Input: part model. Units: mm. Frame: model coordinates. Give positions to 0.01 mm unless a question says otherwise; leave off trailing zeros. Loops run counter-clockwise (first coordinate to the right, second up) from the corner with the lowest first, then second, coordinate; pieces in that order, holes last. Notation, with made-up numbers: (-5, 65.5) -> (47, 65.5) arc R24 ccw to (47, 104.5) -> close; hole circle Ø2 at (34.25, 36.25). An arc over 180 degrees is marked (long way). Answer as a JSON object with one key per item and string values.
Autodesk Inventor part; units mm, degrees
ref_plane "YZ Plane" through (0, 0, 0) normal (1, 0, 0) x (0, 1, 0)
ref_plane "XZ Plane" through (0, 0, 0) normal (0, 1, 0) x (-1, 0, 0)
ref_plane "XY Plane" through (0, 0, 0) normal (0, 0, 1) x (1, 0, 0)
sketch "Sketch1" plane through (0, 0, 0) normal (0, 1, 0) x (-1, 0, 0)
  line L0 (0, 0) -> (7.5, 0)
  line L1 (7.5, -18) -> (0, -18)
  line L2 (0, -18) -> (0, 0)
  arc A0 (7.5, -5) -> (7.5, -13) centre (7.5, -9) ccw
  line L3 (7.5, -18) -> (7.5, -13)
  line L4 (7.5, -5) -> (7.5, 0)
  dimension "d0" = 7.5
  dimension "d1" = 18
  dimension "d5" = 4
  dimension "d6" = 0
  dimension "d7" = 5
  dimension "d8" = 0
extrude "Extrusion2" add sketch "Sketch1" along normal blind 16
properties part number "Lower Base Bearing Holder" material "Brass, Soft Yellow"
Q1. Section D-D, the plane x = -7. Return the cut outline in (y, z), then the cut area to 3 significant figures.
Evaluation:
{"outline": "(0, -18) -> (16, -18) -> (16, -12.97) -> (0, -12.97) -> close; (0, -5.03) -> (16, -5.03) -> (16, 0) -> (0, 0) -> close", "area": "161 mm2"}
Q2. Draft query along Z for faces 1 (the cylindrical face through (-3.5, 7.9, -9.1)), 2 (the flat face through (-7.5, 8, -3)), 3 (the flat face through (-4, 8, -18)). Return one class per face: +Z half, -Z half, draft (parallel to the pull), parting line (faces both ways), or undercut.
Evaluation:
{"face 1": "undercut", "face 2": "draft", "face 3": "-Z half"}
Q3. Pin query (flat end, axial travel): pin 1 (4 mm diameter, centred on y = 3.5, z = -8.5, fed in from -X). Return the tip coordinate at first contact, or that it passes through.
Evaluation:
{"pin 1": "stops at x = -4.38"}
Q4. Section A-A, the plane x = -5.25. Return the cut outline in (y, z).
Evaluation:
{"outline": "(0, -18) -> (16, -18) -> (16, -12.31) -> (0, -12.31) -> close; (0, -5.69) -> (16, -5.69) -> (16, 0) -> (0, 0) -> close"}
Q5. Section C-C, the plane z = -9. Return the cut outline in (x, y).
Evaluation:
{"outline": "(-3.5, 0) -> (0, 0) -> (0, 16) -> (-3.5, 16) -> close"}
Q6. Section B-B, the plane y = 9.5. Return the cut outline in (x, z), then the cut area to 3 significant figures.
Evaluation:
{"outline": "(-7.5, -18) -> (0, -18) -> (0, 0) -> (-7.5, 0) -> (-7.5, -5) arc R4 cw to (-7.5, -13) -> close", "area": "110 mm2"}
Q7. Ray query, line 1 along Z through (x, y) = (-6.5, 13.75); line 2 along X through (y, z) = (9.5, -8.75); line 3 along Z through (x, y) = (-5.25, 7.5). Return the intervals inside material, ascending.
Evaluation:
{"line 1": "z = -18 to -12.87, -5.13 to 0", "line 2": "x = -3.51 to 0", "line 3": "z = -18 to -12.31, -5.69 to 0"}
